Can you work these out from the model? Positions are in its coordinate system, mm. Face numbers are marked on the shaded views. A direction names the side the tool comes from. Give positions to 0.01 mm unless a question says otherwise; leave off trailing zeros. Loops run counter-clockwise (first coordinate to the right, second up) from the corner with the lowest first, then second, coordinate; pieces in that order, holes last. Notation, with made-up numbers: M 28,28.5 L 68,28.5 A20 cw 68,60.5 Z; hole C -6.5,49.25 d3. An arc over 180 degrees is marked long. Put each result on its own line as item: value. Start each with the question number.
1) Imagine slicing it at B-B (x = 12.75). Write out the boundary of the cut face in (y, z) (3 decimals).
2) Please list where these lines run through material, in increasing order: line 1 along X through (y, z) = (30, 13) (3 decimals); line 2 along Y through (x, z) = (14.25, 0); line 3 along Z through (x, y) = (6.25, 48) (3 decimals). Write a range as from..to.
3) If we mould it in two halves opening along X, with no side actions, what happens to the marked faces 1, 2 and 3? For each: +X half, -X half, draft (parallel to the pull), parting line (faces both ways), or undercut.
4) For P1, Ø5, axis at x = 3.5, y = 47.5, coming from the +Z side; P2, Ø5, axis at x = 10.5, y = 34.5, coming from the +Z side (3 decimals); P3, Ø11, axis at x = 12, z = -16, coming from the +Y side; P4, Ø6.5, axis at x = 9.525, z = -18.175, coming from the -Y side, each with a flat end and sliding along its axis, tell me the tip position at first contact or that it passes through.
5) Imagine slicing it at A-A (z = 0). Write out the boundary of the cut face in (x, y), then the cut area to 3 significant figures.
6) Imagine slicing it at D-D (z = 7.5). Write out the boundary of the cut face in (x, y).
7) Imagine slicing it at C-C (y = 47). Write out the boundary of the cut face in (x, z) (3 decimals), then the cut area to 3 significant figures.
8) For the marked faces 4, 5 and 6, which set-ups out of +Z, -Z, +X, -X, +Y, -Y let a thin tool reach every point of the face, with its end or its side?
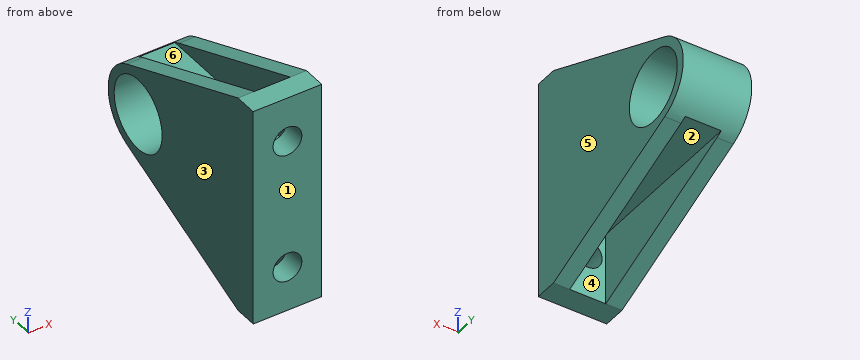
from build123d import *

# Parameters (mm, degrees)
SKETCH1_R           = 10
BOSS_EXTRUDE1_DEPTH = 19.05
SKETCH2_R           = 4
CUT_EXTRUDE1_DEPTH  = 83.63609118
CUT_EXTRUDE2_DEPTH  = 5


with BuildPart() as part:
    # Sketch1 → Boss-Extrude1 (new body)
    with BuildSketch(Plane(origin=(0, 0, 0), x_dir=(0, 0, -1), z_dir=(1, 0, 0))):
        with BuildLine():
            Line((-30.675, 0), (-30.675, 6.35))
            Line((-30.675, 6.35), (-11.55788149, 52.76081668))
            ThreePointArc((-11.55788149, 52.76081668), (0, 60.5), (11.55788149, 52.76081668))
            Line((11.55788149, 52.76081668), (30.675, 6.35))
            Line((30.675, 6.35), (30.675, 0))
            Line((30.675, 0), (-30.675, 0))
        make_face()
        with Locations(Location((0, 48, 0), (0, 0, 180))):
            Circle(SKETCH1_R, mode=Mode.SUBTRACT)
    extrude(amount=BOSS_EXTRUDE1_DEPTH)

    # Sketch2 → Cut-Extrude1 (cut, symmetric)
    with BuildSketch(Plane(origin=(0, 0, 0), x_dir=(1, 0, 0), z_dir=(0, 1, 0))):
        with Locations(Location((9.525, -18.175, 0), (0, 0, 270))):
            Circle(SKETCH2_R)
        with Locations(Location((9.525, 18.175, 0), (0, 0, 270))):
            Circle(SKETCH2_R)
    extrude(amount=CUT_EXTRUDE1_DEPTH, both=True, mode=Mode.SUBTRACT)

    # Sketch3 → Cut-Extrude2 (cut, symmetric)
    with BuildSketch(Plane(origin=(9.525, 0, 0), x_dir=(0, 0, -1), z_dir=(1, 0, 0))):
        Polygon((-10.675, 54.904196759), (-10.675, 6.35), (-30.675, 6.35), align=None)
        Polygon((10.675, 54.904196759), (30.675, 6.35), (10.675, 6.35), align=None)
    extrude(amount=CUT_EXTRUDE2_DEPTH, both=True, mode=Mode.SUBTRACT)


solid = part.part
Recorded:
1. outline: M 0,-30.675 L 6.35,-30.675 L 6.35,-20.541 L 0,-20.541 Z; M 0,-15.809 L 6.35,-15.809 L 6.35,-10.675 L 54.503,-10.675 A12.5 ccw 54.503,10.675 L 6.35,10.675 L 6.35,15.809 L 0,15.809 Z; M 0,20.541 L 6.35,20.541 L 6.35,30.675 L 0,30.675 Z; hole C 48,0 d20
2. line 1: 0..4.525, 14.525..19.05
2. line 2: 0..38, 58..60.5
2. line 3: -10.675..-10, 10..10.675
3. face 1: draft
3. face 2: undercut
3. face 3: -X half
4. P1: z = 14.75
4. P2: z = 10.675
4. P3: y = 54.78
4. P4: through
5. outline: M 0,0 L 19.05,0 L 19.05,38 L 0,38 Z; M 0,58 L 19.05,58 L 19.05,60.5 L 0,60.5 Z
5. area: 772 mm²
6. outline: M 0,0 L 19.05,0 L 19.05,41.39 L 0,41.39 Z; M 0,54.61 L 19.05,54.61 L 19.05,58 L 0,58 Z
7. outline: M 0,-13.931 L 4.525,-13.931 L 4.525,-10.675 L 14.525,-10.675 L 14.525,-13.931 L 19.05,-13.931 L 19.05,-9.95 L 0,-9.95 Z; M 0,9.95 L 19.05,9.95 L 19.05,13.931 L 14.525,13.931 L 14.525,10.675 L 4.525,10.675 L 4.525,13.931 L 0,13.931 Z
7. area: 86.6 mm²
8. face 4: -Z, +Y
8. face 5: +Z, -Z, +X, +Y, -Y
8. face 6: +Z, +Y
